Could you check a few things on this model? Use its own coordinates, in mm. A direction names the side the tool comes from. Give positions to 0.01 mm unless a question says otherwise; leave off trailing zeros. Write each loop counter-clockwise with the first axis right and the second up, starting at its lowest first coordinate (ties: lowest second). Pieces come first, ordered by that corner, then holes. Notation, with made-up numbers: M -10.5,18 L 4.5,18 A16 ccw 4.5,33 Z; hole C 80.25,-21 d4. An arc over 180 degrees is marked long. One line per item, written item: value.
```python
from build123d import *

# Parameters (mm, degrees)
F1_DEPTH = 63.5
F2_R     = 31.5105933146
F3_DEPTH = 63.5
F4_R     = 17.5276637919
F5_DEPTH = 25.4
F7_DEPTH = 50.8


with BuildPart() as f1:
    # F0 (on Front) → F1 (new body)
    with BuildSketch(Plane.XZ):
        Polygon((18.2524688239, -31.795136659), (36.6616304755, -0.0904666463), (18.4091616516, 31.7046700128), (-18.2524688239, 31.795136659), (-36.6616304755, 0.0904666463), (-18.4091616516, -31.7046700128), align=None)
    extrude(amount=F1_DEPTH)

    # F2 (on face) → F3 (join)
    with BuildSketch(Plane(origin=(0, 0, 0), x_dir=(-1, 0, 0), z_dir=(0, 1, 0))):
        Circle(F2_R)
    extrude(amount=F3_DEPTH)

    # F4 (on face) → F5 (join)
    with BuildSketch(Plane(origin=(0.0783464139, 0, 31.7499033359), x_dir=(0.9999969555, 0, -0.0024676036), z_dir=(0.0024676036, 0, 0.9999969555))):
        with Locations((0, -31.75)):
            Circle(F4_R)
    extrude(amount=F5_DEPTH)

    # F6 (on face) → F7 (join)
    with BuildSketch(Plane(origin=(0.141023545, 0, 57.1498260046), x_dir=(0.9999969555, 0, -0.0024676036), z_dir=(0.0024676036, 0, 0.9999969555))):
        Polygon((14.8922465929, -56.5634329038), (28.9351865462, -31.2596525831), (14.0429399534, -6.4462196793), (-14.8922465929, -6.9365670962), (-28.9351865462, -32.2403474169), (-14.0429399534, -57.0537803207), align=None)
    extrude(amount=F7_DEPTH)


solid = f1.part
```
1) If we section it at B-B, the plane z = 22: Write out the boundary of the cut face in (x, y), then the cut area to 3 significant figures.
Outcome:
outline: M -23.94,-63.5 L 23.98,-63.5 L 23.98,0 L 22.56,0 L 22.56,63.5 L -22.56,63.5 L -22.56,0 L -23.94,0 Z
area: 5,910 mm^2
2) If we section it at A-A, the plane x = -24.5: Write out the boundary of the cut face in (y, z).
Outcome:
outline: M -63.5,-21.09 L 0,-21.09 L 0,-19.82 L 63.5,-19.82 L 63.5,19.82 L 0,19.82 L 0,21.04 L -63.5,21.04 Z; M -39.4,57.21 L -24.5,57.21 L -24.73,108.01 L -39.19,108.01 Z
3) I'm going to push flat-ended pins straight in: pin 1 (8 mm diameter, centred on y = 24.5, z = -0.5, fed in from +X); pin 2 (3 mm diameter, centred on x = -6, z = 93.5, fed in from -Y); pin 3 (10 mm diameter, centred on x = -14, y = 10.5, fed in from +Z). Where does each tip first touch, or does it pass through?
Outcome:
pin 1: stops at x = 31.51
pin 2: stops at y = -56.95
pin 3: stops at z = 30.2
4) Please list where these lines run through material, in increasing order: L1, parallel to Z at x = 17.5, y = -36; L2, parallel to Z at x = -14.5, y = -51.5; L3, parallel to Z at x = 0, y = 7.5. Write a range as from..to.
Outcome:
L1: z = -31.79..31.71, 57.11..107.91
L2: z = -31.71..31.79, 57.19..107.99
L3: z = -31.51..31.51
5) If we section it at D-D, the plane z = 78: Write out the boundary of the cut face in (x, y), then the cut area to 3 significant figures.
Outcome:
outline: M -28.74,-32.24 L -13.85,-57.05 L 15.08,-56.56 L 29.13,-31.26 L 14.24,-6.45 L -14.7,-6.94 Z
area: 2,180 mm^2
6) On a 3-axis mill with a long thin cutter (end or side, diameter ignored), from which of +Z, -Z, +X, -X, +Y, -Y can I reach the whole of each face in a straight line? I mean faces 1 (the face through (32, 0, 0)), 2 (the face through (27.33, -31.31, -16.16)), 3 (the face through (27.663, -31.306, 15.585)), 4 (the face through (-1, -63.5, 0)), 5 (the face through (-3.69, -48.86, 44.28)). Say none if no direction works.
Outcome:
face 1: +Y
face 2: -Z, +X, +Y, -Y
face 3: +X, +Y, -Y
face 4: +Z, -Z, +X, -X, -Y
face 5: none
7) If we section it at C-C, the plane y = 20.5: Write out the boundary of the cut face in (x, z), then the cut area to 3 significant figures.
Outcome:
outline: C 0,0 d63.02
area: 3,120 mm^2
